from build123d import *

# Parameters (mm, degrees)
F1_DEPTH = 25.4
F3_R     = 4.8121462922
F4_DEPTH = 50.8
F6_R     = 4.8597300297
F7_DEPTH = 25.4
F8_R     = 3.348410215
F9_DEPTH = 7.62


with BuildPart() as f1:
    # F0 (on Front) → F1 (new body)
    with BuildSketch(Plane.XZ):
        Polygon((-22.5596427917, 14.7743310452), (-22.5596427917, -10.6256689548), (15.5403572083, -10.6256689548), (15.5403572083, 2.0743310452), (28.2403572083, 2.0743310452), (28.2403572083, 14.7743310452), align=None)
    extrude(amount=F1_DEPTH)

    # F3 (on offset) → F4 (cut)
    with BuildSketch(Plane.YZ.offset(9.6647944301)):
        with Locations((-12.7, 7.1543310452)):
            Circle(F3_R)
    extrude(amount=-F4_DEPTH, mode=Mode.SUBTRACT)

    # F6 (on offset) → F7 (cut)
    with BuildSketch(Plane.XY.offset(11.9803310452)):
        with Locations((4.8589497015, -13.0971787283)):
            Circle(F6_R)
    extrude(amount=-F7_DEPTH, mode=Mode.SUBTRACT)

    # F8 (on face) → F9 (cut)
    with BuildSketch(Plane.XY.offset(14.7743310452)):
        with Locations((-10.1922675967, -12.7)):
            Circle(F8_R)
    extrude(amount=-F9_DEPTH, mode=Mode.SUBTRACT)


solid = f1.part
Design review of the part built by this model. Coordinates are the model's own, in mm. A direction names the side the tool comes from. Round coordinates to 2 decimals unless told otherwise and drop trailing zeros. Order: outer loops, then holes, each group sorted by start corner. A loop starts at its lowest first (then second) coordinate and runs counter-clockwise, first axis right, second up.
1) For L1, parallel to Z at x = -20, y = -12.75; L2, parallel to Y at x = 5, z = -0.75; L3, parallel to X at y = -12.7, z = 12.9, list the stretches that pass through material, from the lowest coordinate up.
The answers:
L1: z = -10.63 to 2.34, 11.97 to 14.77
L2: y = -25.4 to -17.95, -8.24 to 0
L3: x = -22.56 to -13.54, -6.84 to 28.24
2) Draft analysis for pull direction X (two halves, no side actions). For faces 6 (the flat face through (2, -25.4, 2)), 7 (the flat face through (15.54, -13, -4)), 8 (the flat face through (5, -13, 11.98)), state which applies: released by +X, released by -X, zero draft, split by the parting line, or undercut.
The answers:
face 6: zero draft
face 7: released by +X
face 8: undercut
3) Consider section C-C (z = 6). State the section outline as (x, y) points.
The answers:
outline: (-22.56, -25.4) - (28.24, -25.4) - (28.24, 0) - (-22.56, 0) - (-22.56, -8.03) - (9.66, -8.03) - (9.66, -12.38) arc R4.86 cw to (9.66, -13.82) - (9.66, -17.37) - (7.17, -17.37) arc R4.86 cw to (2.55, -17.37) - (-22.56, -17.37) - close
4) Consider section B-B (z = -5.25). State the section outline as (x, y) points, plus the area to 3 significant figures.
The answers:
outline: (-22.56, -25.4) - (15.54, -25.4) - (15.54, 0) - (-22.56, 0) - close; hole circle Ø9.72 at (4.86, -13.1)
area: 894 mm2
5) Consider section D-D (y = -6.75). State the section outline as (x, z) points.
The answers:
outline: (-22.56, -10.63) - (15.54, -10.63) - (15.54, 2.07) - (28.24, 2.07) - (28.24, 14.77) - (-22.56, 14.77) - close
6) Machinability: for faces 1 (the flat face through (9.665, -11, 7)), 2 (the flat face through (22, -13, 2.074)), 3 (the flat face through (-22.56, -13, 2)), 4 (the cylindrical face through (3.805, -17.841, -1.676)), 5 (the cylindrical face through (-8.65, -15.67, 13.18)), which of the approach directions +Z, -Z, +X, -X, +Y, -Y give a long, thin tool a straight path to every point of the face, cutting with its end or side? Answer none if there is none.
The answers:
face 1: -X
face 2: -Z, +X, +Y, -Y
face 3: +Z, -Z, -X, +Y, -Y
face 4: -Z
face 5: +Z
7) Consider section A-A (y = -15.5). State the section outline as (x, z) points, plus the area to 3 significant figures.
The answers:
outline: (-22.56, -10.63) - (0.63, -10.63) - (0.63, 3.24) - (-22.56, 3.24) - close; (-22.56, 11.07) - (-12.03, 11.07) - (-12.03, 14.77) - (-22.56, 14.77) - close; (-8.36, 11.07) - (0.63, 11.07) - (0.63, 11.98) - (9.08, 11.98) - (9.08, 11.07) - (9.66, 11.07) - (9.66, 3.24) - (9.08, 3.24) - (9.08, -10.63) - (15.54, -10.63) - (15.54, 2.07) - (28.24, 2.07) - (28.24, 14.77) - (-8.36, 14.77) - close
area: 738 mm2
8) Clearance check with flat-ended pins moving along their axes: pin 1 Ø10 at (x, y) = (23, -14.5) entering from -Z; pin 2 Ø6.5 at (y, z) = (-7.5, -5.5) entering from +X; pin 3 Ø5.5 at (x, y) = (-10.19, -12.7) entering from +Z. State where each tip first meets the part, or that it passes through.
The answers:
pin 1: stops at z = 2.07
pin 2: stops at x = 15.54
pin 3: stops at z = 3.21
